Check sheet for the drawn part. Datum: minimum x, y, z corner. Units: mm. A direction names the side the tool comes from. Round coordinates to 2 decimals unless told otherwise and drop trailing zeros. Write each loop counter-clockwise with the first axis right and the second up, starting at its lowest first coordinate (ties: lowest second). Pieces come first, ordered by that corner, then holes.
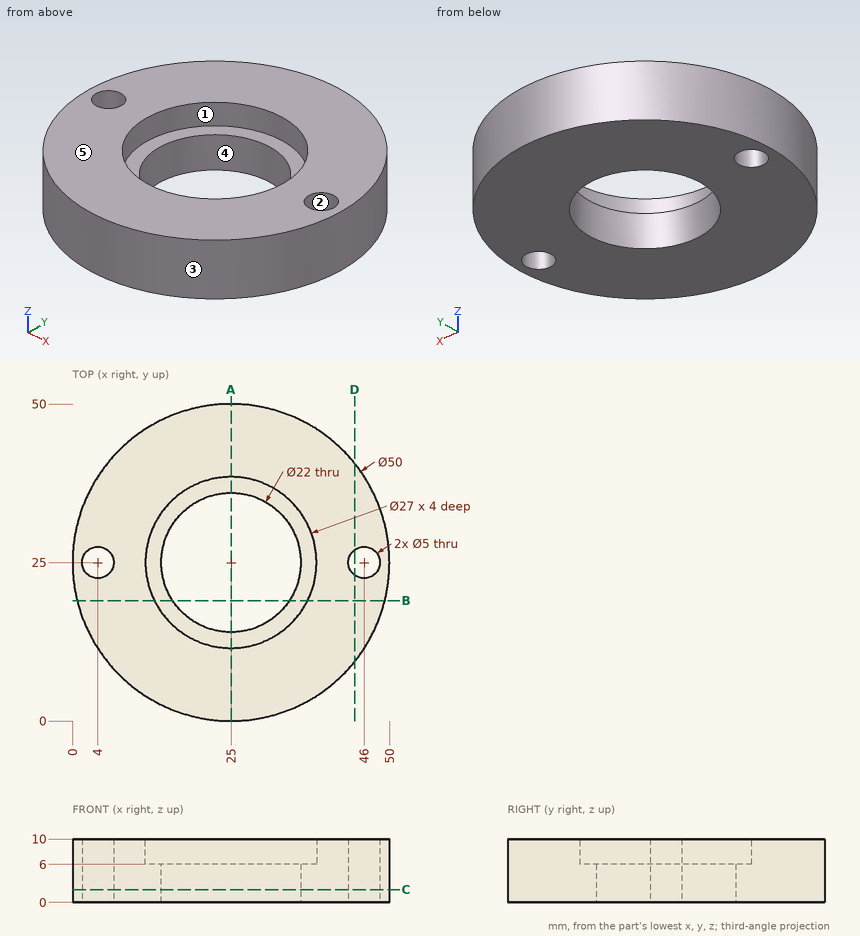
Q1. Sectioned sample at D-D (x = 44.5). Enter the section's corners in (y, z).
Recorded:
outline: (9.36, 0) - (23, 0) - (23, 10) - (9.36, 10) - close; (27, 0) - (40.64, 0) - (40.64, 10) - (27, 10) - close
Q2. Material ranges on line 1 along Y through (x, z) = (25, 4.75); line 2 along Y through (x, z) = (25, 7.4); line 3 along X through (y, z) = (33, 4), recorded low to high.
Recorded:
line 1: y = 0 to 14, 36 to 50
line 2: y = 0 to 11.5, 38.5 to 50
line 3: x = 1.31 to 17.45, 32.55 to 48.69
Q3. Tool access check on the marked faces 1 and 2. Record the directions out of +Z, -Z, +X, -X, +Y, -Y that give a thin tool (end or side, any length) a straight path to the whole face; none if there is none.
Recorded:
face 1: +Z
face 2: +Z, -Z
Q4. Sectioned sample at A-A (x = 25). Enter the section's corners in (y, z).
Recorded:
outline: (0, 0) - (14, 0) - (14, 6) - (11.5, 6) - (11.5, 10) - (0, 10) - close; (36, 0) - (50, 0) - (50, 10) - (38.5, 10) - (38.5, 6) - (36, 6) - close
Q5. Depth check by flat-ended pin: P1, Ø3, axis at x = 35.5, z = 4, coming from the -Y side; P2, Ø1.5, axis at y = 29, z = 6.5, coming from the +X side; P3, Ø3, axis at y = 37.5, z = 8, coming from the -X side. Enter the tip coordinate at first touch or a pass-through.
Recorded:
P1: stops at y = 1.68
P2: stops at x = 49.79
P3: stops at x = 2.55
Q6. Sectioned sample at B-B (y = 19). Enter the section's corners in (x, z), plus the area to 3 significant figures.
Recorded:
outline: (0.73, 0) - (15.78, 0) - (15.78, 6) - (12.91, 6) - (12.91, 10) - (0.73, 10) - close; (34.22, 0) - (49.27, 0) - (49.27, 10) - (37.09, 10) - (37.09, 6) - (34.22, 6) - close
area: 278 mm2
Q7. Sectioned sample at C-C (z = 2). Enter the section's corners in (x, y), plus the area to 3 significant figures.
Recorded:
outline: circle Ø50 at (25, 25); hole circle Ø5 at (4, 25); hole circle Ø22 at (25, 25); hole circle Ø5 at (46, 25)
area: 1,540 mm2
Q8. Release check for a two-part mould opening along X. For the marked faces 3, 4 and 5 record: released by +X, released by -X, zero draft, split by the parting line, or undercut.
Recorded:
face 3: split by the parting line
face 4: undercut
face 5: zero draft
